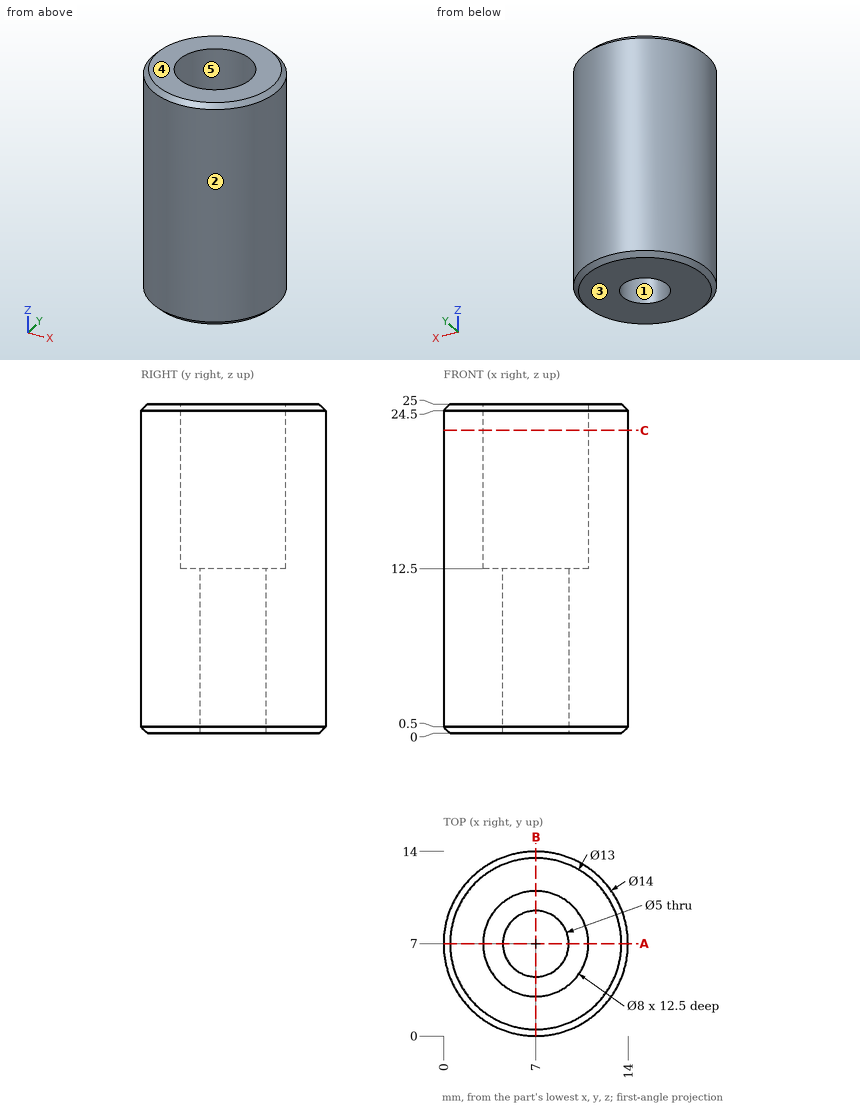
Job drawing, mm, ordinate dimensions from the low corner. One solid piece. A direction names the side the tool comes from. Round coordinates to 2 decimals unless told otherwise and drop trailing zeros. Order: outer loops, then holes, each group sorted by start corner. A loop starts at its lowest first (then second) coordinate and runs counter-clockwise, first axis right, second up. Notation, with made-up numbers: (60, 28.25) -> (71, 28.25) arc R33 ccw to (71, 63.25) -> close; hole circle Ø8 at (-14.75, 56.25). An arc over 180 degrees is marked (long way). Answer in a Markdown table with one row per item.
1) Pin check, flat tips, straight feed: P1, Ø6, axis at x = 3.5, z = 21.5, coming from the +Y side; P2, Ø4, axis at x = 12.5, z = 19, coming from the +Y side; P3, Ø4, axis at x = 6, y = 5.5, coming from the +Z side. Stop position of each tip, or through.
Values:
| item | result |
|---|---|
| P1 | y = 13.98 |
| P2 | y = 13.06 |
| P3 | z = 12.5 |
2) Mould opens along Y. For the marked faces 1, 2 and 3 say: released by +Y, released by -Y, zero draft, split by the parting line, or undercut.
Values:
| item | result |
|---|---|
| face 1 | undercut |
| face 2 | split by the parting line |
| face 3 | zero draft |
3) Band-saw the part on C-C on z = 23. Give the cut face in (x, y), and give its area (3 significant figures).
Values:
| item | result |
|---|---|
| outline | circle Ø14 at (7, 7); hole circle Ø8 at (7, 7) |
| area | 104 mm2 |
4) Band-saw the part on A-A on y = 7. Give the cut face in (x, z), and give its area (3 significant figures).
Values:
| item | result |
|---|---|
| outline | (0, 0.5) -> (0.5, 0) -> (4.5, 0) -> (4.5, 12.5) -> (3, 12.5) -> (3, 25) -> (0.5, 25) -> (0, 24.5) -> close; (9.5, 0) -> (13.5, 0) -> (14, 0.5) -> (14, 24.5) -> (13.5, 25) -> (11, 25) -> (11, 12.5) -> (9.5, 12.5) -> close |
| area | 187 mm2 |
5) Wall check: L1, parallel to Y at x = 7, z = 2.75; L2, parallel to Z at x = 9, y = 9.5; L3, parallel to X at y = 5.5, z = 16.5. Give the ranges that are in metal, low to high.
Values:
| item | result |
|---|---|
| L1 | 0 to 4.5, 9.5 to 14 |
| L2 | 0 to 12.5 |
| L3 | 0.16 to 3.29, 10.71 to 13.84 |
6) Which spindle directions (+Z, -Z, +X, -X, +Y, -Y) get a long thin tool onto all of the face, cutting with end or side? Do the marked faces 4 and 5. Say none if no direction does.
Values:
| item | result |
|---|---|
| face 4 | +Z, +X, -X, +Y, -Y |
| face 5 | +Z |
